Check sheet for the modelled part. Datum: model origin and axes. Units: mm. A direction names the side the tool comes from. Give positions to 0.01 mm unless a question says otherwise; leave off trailing zeros. Loops run counter-clockwise (first coordinate to the right, second up) from the corner with the lowest first, then second, coordinate; pieces in that order, holes last. Notation, with made-up numbers: (-38, -32) - (-11, -32) arc R29 cw to (-11, -3) - close; hole circle Ø10 at (46.25, 24). An arc over 180 degrees is marked (long way). Use CSV: the item, a comma, the result in double quotes.
from build123d import *

# Parameters (mm, degrees)
SKETCH2_W                        = 4.7625
SKETCH2_H                        = 19.05
BOSS_EXTRUDE1_DEPTH              = 20.955
BOSS_EXTRUDE1_2_DEPTH            = 20.955
SKETCH3_W                        = 25.4
SKETCH3_H                        = 15.875
BOSS_EXTRUDE2_DEPTH              = 22.225
SKETCH2_3_W                      = 14.2875
SKETCH2_3_H                      = 19.05
SKETCH2_3_W_2                    = 4.7625
BOSS_EXTRUDE3_DEPTH              = 6.35
FILLET1_R                        = 9.525
F_12_0MM_DOWEL_HOLE1_D           = 12
F_12_0MM_DOWEL_HOLE1_CSINK_D     = 12.05
F_12_0MM_DOWEL_HOLE1_CSINK_ANGLE = 90
FILLET2_R                        = 1.905
SKETCH5_W                        = 9.525
SKETCH5_H                        = 12.7
CUT_EXTRUDE1_DEPTH               = 41.907013457


with BuildPart() as part:
    # Sketch2 → Boss-Extrude1 (new body)
    with BuildSketch(Plane(origin=(0, 0, 0), x_dir=(1, 0, 0), z_dir=(0, 1, 0))):
        with Locations((2.38125, 9.525)):
            Rectangle(SKETCH2_W, SKETCH2_H)
    extrude(amount=BOSS_EXTRUDE1_DEPTH)



with BuildPart() as body_2:
    # Sketch2 → Boss-Extrude1 2 (new body)
    with BuildSketch(Plane(origin=(0, 0, 0), x_dir=(1, 0, 0), z_dir=(0, 1, 0))):
        with Locations((21.43125, 9.525)):
            Rectangle(SKETCH2_W, SKETCH2_H)
    extrude(amount=BOSS_EXTRUDE1_2_DEPTH)


with BuildPart() as part_1:
    add(part.part)

    add(body_2.part)  # Boss-Extrude2 merges body 2
    # Sketch3 → Boss-Extrude2 (add)
    with BuildSketch(Plane(origin=(0, 0, 0), x_dir=(1, 0, 0), z_dir=(0, 1, 0))):
        with Locations((14.2875, 9.525)):
            Rectangle(SKETCH3_W, SKETCH3_H)
    extrude(amount=-BOSS_EXTRUDE2_DEPTH)

    # Sketch2<3> → Boss-Extrude3 (add)
    with BuildSketch(Plane(origin=(0, 0, 0), x_dir=(1, 0, 0), z_dir=(0, 1, 0))):
        with Locations((11.90625, 9.525)):
            Rectangle(SKETCH2_3_W, SKETCH2_3_H)
        with Locations((26.19375, 9.525)):
            Rectangle(SKETCH2_3_W_2, SKETCH2_3_H)
        with Locations((2.38125, 9.525)):
            Rectangle(SKETCH2_3_W_2, SKETCH2_3_H)
        with Locations((21.43125, 9.525)):
            Rectangle(SKETCH2_3_W_2, SKETCH2_3_H)
    extrude(amount=-BOSS_EXTRUDE3_DEPTH)

    # Fillet1
    fillet1_edges = [part_1.edges().sort_by_distance(p)[0] for p in [
        (2.38125, 20.955, -19.05),
        (2.38125, 20.955, 0),
        (21.43125, 20.955, 0),
        (21.43125, 20.955, -19.05),
    ]]
    fillet(fillet1_edges, radius=FILLET1_R - 0.0001)  # a hair under: the kernel refuses the full size

    # Ø12.0mm Dowel Hole1 (through all)
    with Locations(Plane(origin=(0, 11.43, -9.525), x_dir=(0, 0, -1), z_dir=(-1, 0, 0))):
        with Locations((0, 0)):
            CounterSinkHole(F_12_0MM_DOWEL_HOLE1_D / 2, F_12_0MM_DOWEL_HOLE1_CSINK_D / 2, counter_sink_angle=F_12_0MM_DOWEL_HOLE1_CSINK_ANGLE)

    # Fillet2
    fillet2_edges = [part_1.edges().sort_by_distance(p)[0] for p in [
        (1.5875, -14.2875, -1.5875),
        (1.5875, -14.2875, -17.4625),
        (26.9875, -14.2875, -17.4625),
        (26.9875, -14.2875, -1.5875),
    ]]
    fillet(fillet2_edges, radius=FILLET2_R)

    # Sketch5 → Cut-Extrude1 (cut, through all)
    with BuildSketch(Plane(origin=(0, 0, 0), x_dir=(1, 0, 0), z_dir=(0, 1, 0))):
        with Locations((14.2875, 9.525)):
            Rectangle(SKETCH5_W, SKETCH5_H)
    extrude(amount=-CUT_EXTRUDE1_DEPTH, mode=Mode.SUBTRACT)


solid = part_1.part
1. Go/stop test with flat-tipped pins: pin 1 Ø1.5 at (x, y) = (18, -14.5) entering from +Z; pin 2 Ø6 at (x, z) = (22.5, -3) entering from +Y; pin 3 Ø3 at (x, z) = (15.5, -15) entering from +Y. Record where each tip stops, or that it passes through.
Completed:
pin 1,"stops at z = -1.59"
pin 2,"stops at y = 20.28"
pin 3,"stops at y = 0"
2. Scan lines: line 1 along X through (y, z) = (-1.5, -7.5) (3 decimals); line 2 along X through (y, z) = (-14, -15.75) (3 decimals); line 3 along Z through (x, y) = (4.25, 9). Record each from-to range of solid material in increasing order.
Completed:
line 1,"x = 0 to 9.525, 19.05 to 28.575"
line 2,"x = 1.597 to 9.525, 19.05 to 26.978"
line 3,"z = -19.05 to -15.01, -4.04 to 0"
3. Release check for a two-part mould opening along Y. For faces 5 (the face through (21.46, 9.63, -3.8)), 6 (the face through (9.525, -11, -9)), 7 (the face through (8, -22.225, -10)) record: released by +Y, released by -Y, zero draft, split by the parting line, or undercut.
Completed:
face 5,"undercut"
face 6,"zero draft"
face 7,"released by -Y"
4. Set-up check for faces 1 (the face through (4.762, 5.67, -7.27)), 2 (the face through (14, -14, -17.462)), 3 (the face through (26.444, -14.399, -2.16)), 4 (the face through (26.987, -14, -9)): record each of +Z, -Z, +X, -X, +Y, -Y from which the full face is reachable in a straight line by a thin tool's end or side.
Completed:
face 1,"+Z, -Z, +Y"
face 2,"-Z, +X, -X, -Y"
face 3,"+Z, +X, -Y"
face 4,"+Z, -Z, +X, -Y"
5. Sectioned sample at D-D, the plane y = -3.5. Record the boundary of the cut face in (x, z) (3 decimals), and give its area (3 significant figures).
Completed:
outline,"(0, -19.05) - (28.575, -19.05) - (28.575, 0) - (0, 0) - close; hole (9.525, -15.875) - (19.05, -15.875) - (19.05, -3.175) - (9.525, -3.175) - close"
area,"423 mm²"
